```python
from build123d import *

# Parameters (mm, degrees)
F0_R     = 234.95
F0_R_2   = 13.49375
F0_R_3   = 14.2875
F0_R_4   = 30
F1_DEPTH = 12.7
F2_D     = 6.8
F3_D     = 8.4
F4_D     = 10.3
F5_R     = 295.3741287218
F5_R_2   = 212.725
F6_DEPTH = 4.7625


with BuildPart() as f1:
    # F0 (on Top) → F1 (new body)
    with BuildSketch(Plane.XY):
        Circle(F0_R)
        with Locations((-114.3, -114.3)):
            Circle(F0_R_2, mode=Mode.SUBTRACT)
        with Locations((0, -95.25)):
            Circle(F0_R_3, mode=Mode.SUBTRACT)
        with Locations((114.3, -114.3)):
            Circle(F0_R_2, mode=Mode.SUBTRACT)
        with Locations((-114.3, 114.3)):
            Circle(F0_R_2, mode=Mode.SUBTRACT)
        Circle(F0_R_4, mode=Mode.SUBTRACT)
        with Locations((114.3, 114.3)):
            Circle(F0_R_2, mode=Mode.SUBTRACT)
    extrude(amount=F1_DEPTH)

    # F2 (through all)
    with Locations(Plane(origin=(0, 0, 0), x_dir=(1, 0, 0), z_dir=(0, 0, -1))):
        with Locations((-114.3, 85.725), (-85.725, 114.3), (-142.875, 114.3), (-114.3, 142.875), (-142.875, -114.3), (-114.3, -142.875), (-85.725, -114.3), (-114.3, -85.725), (114.3, -142.875), (142.875, -114.3), (85.725, -114.3), (114.3, -85.725), (85.725, 114.3), (114.3, 85.725), (142.875, 114.3), (114.3, 142.875)):
            Hole(F2_D / 2)

    # F3 (through all)
    with Locations(Plane(origin=(0, 0, 0), x_dir=(1, 0, 0), z_dir=(0, 0, -1))):
        with Locations((-142.875, 19.05), (-142.875, -19.05), (142.875, -19.05), (142.875, 19.05)):
            Hole(F3_D / 2)

    # F4 (through all)
    with Locations(Plane(origin=(0, 0, 0), x_dir=(1, 0, 0), z_dir=(0, 0, -1))):
        with Locations((-55, 55), (-55, -55), (55, -55), (55, 55)):
            Hole(F4_D / 2)

    # F5 (on face) → F6 (cut)
    with BuildSketch(Plane.XY):
        Circle(F5_R)
        Circle(F5_R_2, mode=Mode.SUBTRACT)
    extrude(amount=F6_DEPTH, mode=Mode.SUBTRACT)


solid = f1.part
```
The listing builds one solid part. Answer for the finished solid, in the listing's coordinates (mm). A direction names the side the tool comes from. Give positions to 0.01 mm unless a question says otherwise; leave off trailing zeros. Loops run counter-clockwise (first coordinate to the right, second up) from the corner with the lowest first, then second, coordinate; pieces in that order, holes last. Notation, with made-up numbers: (73.5, 49) - (112.5, 49) arc R11 cw to (112.5, 68) - close; hole circle Ø8 at (18.5, -8.5). An arc over 180 degrees is marked (long way). Return JSON: item names as keys, results as strings. Group by question number.
1. Find section B-B (x = 0). State how many separate pieces and enclosed holes the cut face has, then the cut area to 3 significant figures.
2. Find section D-D (y = -95.25). Write down the section's boundary in (x, z).
3. Determine the mould class of faces 1 (the flat face through (44, 3, 0)), 2 (the cylindrical face through (120.53, 102.33, 6.26)), 3 (the cylindrical face through (-186.45, -142.96, 8.68)), 4 (the cylindrical face through (-59.76, -53.03, 6.44)) for opening direction X: pulls with the +X half, pulls with the -X half, needs draft (parallel to the pull), parting line crosses it, or undercut.
4. Straight lines are drawn through the part: line 1 (Y direction, x = 2, z = 7.5); line 2 (Y direction, x = -8, z = 8.5); line 3 (Z direction, x = -61, y = 212.5). For each, find the intervals that lie inside material, in ascending order. Write a range as [from, to].
5. Given pin 1 Ø3 at (y, z) = (139.5, 1.5) entering from -X; pin 2 Ø5 at (x, y) = (-142.875, 19.05) entering from -Z; pin 3 Ø3 at (y, z) = (-153.5, 9) entering from +X; pin 4 Ø1.5 at (y, z) = (-116, 1.5) entering from +X, each flat-ended and moving along its own axis, determine where each tip first touches the part or whether it passes through.
6. Which of the six approach directions +Z, -Z, +X, -X, +Y, -Y give full straight-line access (tool end or side, diameter ignored) to faces 5 (the cylindrical face through (-29.97, 1.32, 6.26)), 6 (the flat face through (-36, 210, 4.762))?
7. Find section C-C (x = -183.5). Write down the section's boundary in (y, z), then the cut area to 3 significant figures.
Verdict:
{
 "1": {"separate pieces": "3", "enclosed holes": "0", "area": "4,630 mm^2"},
 "2": {"outline": "(-214.78, 4.76) - (-190.21, 4.76) - (-190.21, 0) - (-14.29, 0) - (-14.29, 12.7) - (-214.78, 12.7) - close; (14.29, 0) - (190.21, 0) - (190.21, 4.76) - (214.78, 4.76) - (214.78, 12.7) - (14.29, 12.7) - close"},
 "3": {"face 1": "needs draft", "face 2": "undercut", "face 3": "parting line crosses it", "face 4": "undercut"},
 "4": {"line 1": "y = [-234.94, -109.4], [-81.1, -29.93], [29.93, 234.94]", "line 2": "y = [-234.81, -107.09], [-83.41, -28.91], [28.91, 234.81]", "line 3": "z = [4.76, 12.7]"},
 "5": {"pin 1": "stops at x = -161.89", "pin 2": "passes through", "pin 3": "stops at x = 179.16", "pin 4": "stops at x = 178.8"},
 "6": {"face 5": "+Z, -Z", "face 6": "-Z"},
 "7": {"outline": "(-146.73, 4.76) - (-107.61, 4.76) - (-107.61, 0) - (107.61, 0) - (107.61, 4.76) - (146.73, 4.76) - (146.73, 12.7) - (-146.73, 12.7) - close", "area": "3,350 mm^2"}
}
